Model file for the job. Use its own axes, mm. Round coordinates to 2 decimals unless told otherwise and drop trailing zeros. Loops run counter-clockwise (first coordinate to the right, second up) from the corner with the lowest first, then second, coordinate; pieces in that order, holes last. Notation, with made-up numbers: (86, 23) -> (100, 23) arc R22 cw to (100, 53) -> close; hole circle Ø4 at (53, 58.25). An arc over 180 degrees is marked (long way). Use a Markdown table: item, result.
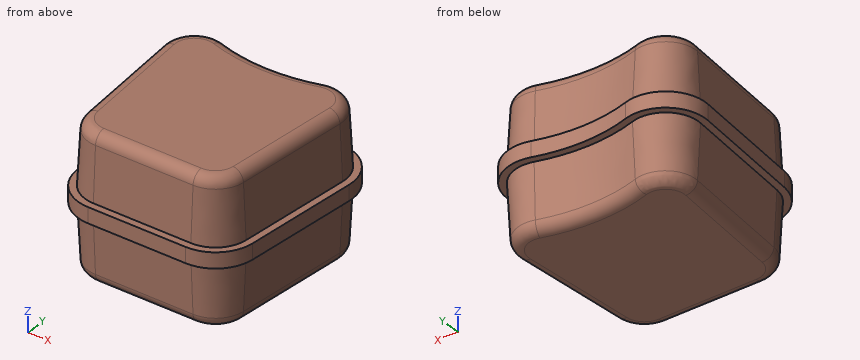
from build123d import *

# Parameters (mm, degrees)
BOSS_EXTRUDE1_DEPTH           = 32.5
BOSS_EXTRUDE1_TAPER           = 3.0000000000000067
BOSS_EXTRUDE1_OTHER_WAY_DEPTH = 32.5
BOSS_EXTRUDE1_OTHER_WAY_TAPER = 3.0000000000000067
FILLET1_R                     = 5
EXTRUDE_THIN1_DEPTH           = 3.5


with BuildPart() as part:
    # Sketch1 → Boss-Extrude1 (new body)
    with BuildSketch(Plane(origin=(0, 0, 0), x_dir=(0, 1, 0), z_dir=(0, 0, 1))):
        with BuildLine():
            ThreePointArc((-39, -22), (-35.05916005215183, -32.13385311423494), (-25.307336141214776, -36.94292047137618))
            Line((-25.307336141214776, -36.94292047137618), (26.697869727868188, -41.49278642925244))
            ThreePointArc((26.697869727868188, -41.49278642925244), (39.67535451570329, -35.97364601503939), (42.33767155756914, -22.124888298230207))
            ThreePointArc((42.33767155756914, -22.124888298230207), (39, 9.18e-15), (42.33767155756914, 22.124888298230207))
            ThreePointArc((42.33767155756914, 22.124888298230207), (39.67535451570329, 35.97364601503939), (26.697869727868188, 41.49278642925244))
            Line((26.697869727868188, 41.49278642925244), (-25.307336141214776, 36.94292047137618))
            ThreePointArc((-25.307336141214776, 36.94292047137618), (-35.059160052151825, 32.13385311423494), (-39, 22))
            Line((-39, 22), (-39, -22))
        make_face()
    extrude(amount=BOSS_EXTRUDE1_DEPTH, taper=BOSS_EXTRUDE1_TAPER)

    # Sketch1 → Boss-Extrude1 other way (add)
    with BuildSketch(Plane(origin=(0, 0, 0), x_dir=(0, 1, 0), z_dir=(0, 0, 1))):
        with BuildLine():
            ThreePointArc((-39, -22), (-35.05916005215183, -32.13385311423494), (-25.307336141214776, -36.94292047137618))
            Line((-25.307336141214776, -36.94292047137618), (26.697869727868188, -41.49278642925244))
            ThreePointArc((26.697869727868188, -41.49278642925244), (39.67535451570329, -35.97364601503939), (42.33767155756914, -22.124888298230207))
            ThreePointArc((42.33767155756914, -22.124888298230207), (39, 9.18e-15), (42.33767155756914, 22.124888298230207))
            ThreePointArc((42.33767155756914, 22.124888298230207), (39.67535451570329, 35.97364601503939), (26.697869727868188, 41.49278642925244))
            Line((26.697869727868188, 41.49278642925244), (-25.307336141214776, 36.94292047137618))
            ThreePointArc((-25.307336141214776, 36.94292047137618), (-35.059160052151825, 32.13385311423494), (-39, 22))
            Line((-39, 22), (-39, -22))
        make_face()
    extrude(amount=-BOSS_EXTRUDE1_OTHER_WAY_DEPTH, taper=BOSS_EXTRUDE1_OTHER_WAY_TAPER)

    # Fillet1
    fillet1_edges = [part.edges().sort_by_distance(p)[0] for p in [
        (30.983152183423496, -33.80339034416901, -32.5),
        (37.52108201484714, 0.8437150585246758, -32.5),
        (34.90357401366931, 38.35020693767984, -32.5),
        (6.661e-14, 37.296747173301156, -32.5),
        (-30.9831521834235, -33.80339034416899, 32.50000000000001),
        (5.09e-15, -37.296747173301156, 32.50000000000001),
        (30.983152183423503, -33.80339034416899, 32.50000000000001),
        (37.521082014847224, 0.8437150585246735, 32.500000000000014),
        (34.9035740136693, 38.35020693767984, 32.50000000000001),
        (-34.903574013669285, 38.35020693767984, -32.5),
        (-8.9e-16, 37.29674717330116, 32.50000000000001),
        (-34.9035740136693, 38.35020693767985, 32.50000000000001),
        (-37.52108201484706, 0.8437150585246949, 32.5),
        (-37.521082014847146, 0.8437150585246864, -32.5),
        (-30.983152183423496, -33.803390344168996, -32.5),
        (1.119e-14, -37.296747173301156, -32.5),
    ]]
    fillet(fillet1_edges, radius=FILLET1_R)

    # Sketch1<2> → Extrude-Thin1 (add, symmetric)
    with BuildSketch(Plane(origin=(0, 0, 0), x_dir=(0, 1, 0), z_dir=(0, 0, 1))):
        with BuildLine():
            Line((-42, -22), (-42, 22))
            ThreePointArc((-42, 21.999999999999996), (-37.270992062582195, 34.160623737081934), (-25.56880336945773, 39.93150456565142))
            Line((-25.56880336945773, 39.93150456565142), (26.436402499625235, 44.48137052352768))
            ThreePointArc((26.436402499625235, 44.48137052352768), (42.009384245027356, 37.858402026472014), (45.20416469526637, 21.239892766301))
            ThreePointArc((45.20416469526637, 21.239892766300997), (42, 8.82e-15), (45.20416469526637, -21.239892766300997))
            ThreePointArc((45.20416469526637, -21.239892766301), (42.009384245027356, -37.858402026472014), (26.436402499625235, -44.48137052352768))
            Line((26.436402499625235, -44.48137052352768), (-25.56880336945773, -39.93150456565142))
            ThreePointArc((-25.568803369457736, -39.931504565651416), (-37.270992062582195, -34.16062373708193), (-42, -22.000000000000004))
        make_face()
        with BuildLine():
            Line((-36, -22), (-36, 22))
            ThreePointArc((-36, 22.000000000000004), (-32.84732804172147, 30.107082491387963), (-25.045868912971823, 33.95433637710095))
            Line((-25.045868912971823, 33.954336377100944), (26.95933695611114, 38.5042023349772))
            ThreePointArc((26.95933695611114, 38.5042023349772), (37.341324786379225, 34.08889000360676), (39.471178419871904, 23.009883830159414))
            ThreePointArc((39.471178419871904, 23.009883830159417), (36, 9.55e-15), (39.471178419871904, -23.009883830159417))
            ThreePointArc((39.471178419871904, -23.009883830159414), (37.341324786379225, -34.08889000360676), (26.95933695611114, -38.5042023349772))
            Line((26.95933695611114, -38.5042023349772), (-25.045868912971823, -33.954336377100944))
            ThreePointArc((-25.045868912971816, -33.95433637710095), (-32.84732804172146, -30.107082491387953), (-36, -21.999999999999996))
        make_face(mode=Mode.SUBTRACT)
    extrude(amount=EXTRUDE_THIN1_DEPTH, both=True)


solid = part.part
Q1. Band-saw the part on B-B, the plane z = -13. Give the cut face in (x, y).
Results list:
| item | result |
|---|---|
| outline | (-40.81, 26.76) -> (-36.26, -25.25) arc R14.32 ccw to (-22, -38.32) -> (22, -38.32) arc R14.32 ccw to (36.26, -25.25) -> (40.81, 26.76) arc R14.32 ccw to (22.33, 41.69) arc R75.68 cw to (-22.33, 41.69) arc R14.32 ccw to start |
Q2. Drill centre lines: L1, parallel to Z at x = -39, y = -2; L2, parallel to X at y = 37.5, z = -20; L3, parallel to X at y = 24, z = -0.5. Where is each one in solid material? Low to high. Write a range as from..to.
Results list:
| item | result |
|---|---|
| L1 | z = -3.5..3.5 |
| L2 | x = -36.77..36.77 |
| L3 | x = -44.27..44.27 |
Q3. Flat gauge pins, fed straight in: pin 1 (6 mm diameter, centred on y = 0.5, z = 16.5, fed in from -X); pin 2 (2 mm diameter, centred on y = 17.5, z = -5.5, fed in from +X); pin 3 (12 mm diameter, centred on x = -18.5, z = 2, fed in from +Y). Where does each tip first touch, or does it go through?
Results list:
| item | result |
|---|---|
| pin 1 | stops at x = -38.64 |
| pin 2 | stops at x = 40.5 |
| pin 3 | stops at y = 45.89 |
Q4. Band-saw the part on A-A, the plane z = -1.5. Give the cut face in (x, y).
Results list:
| item | result |
|---|---|
| outline | (-44.48, 26.44) -> (-39.93, -25.57) arc R18 ccw to (-22, -42) -> (22, -42) arc R18 ccw to (39.93, -25.57) -> (44.48, 26.44) arc R18 ccw to (21.24, 45.2) arc R72 cw to (-21.24, 45.2) arc R18 ccw to start |
